Print and shaded views of the part. All mm, measured from the part's lowest x, y and z. Coordinates: 2 decimals unless noted, no trailing zeros. Order: outer loops, then holes, each group sorted by start corner. A loop starts at its lowest first (then second) coordinate and runs counter-clockwise, first axis right, second up. Notation, with made-up numbers: M -24,4.5 L 23,4.5 A27 cw 23,43.5 Z; hole C 2.25,9 d5. An arc over 180 degrees is marked long. Return JSON: item names as keys, results as strings.
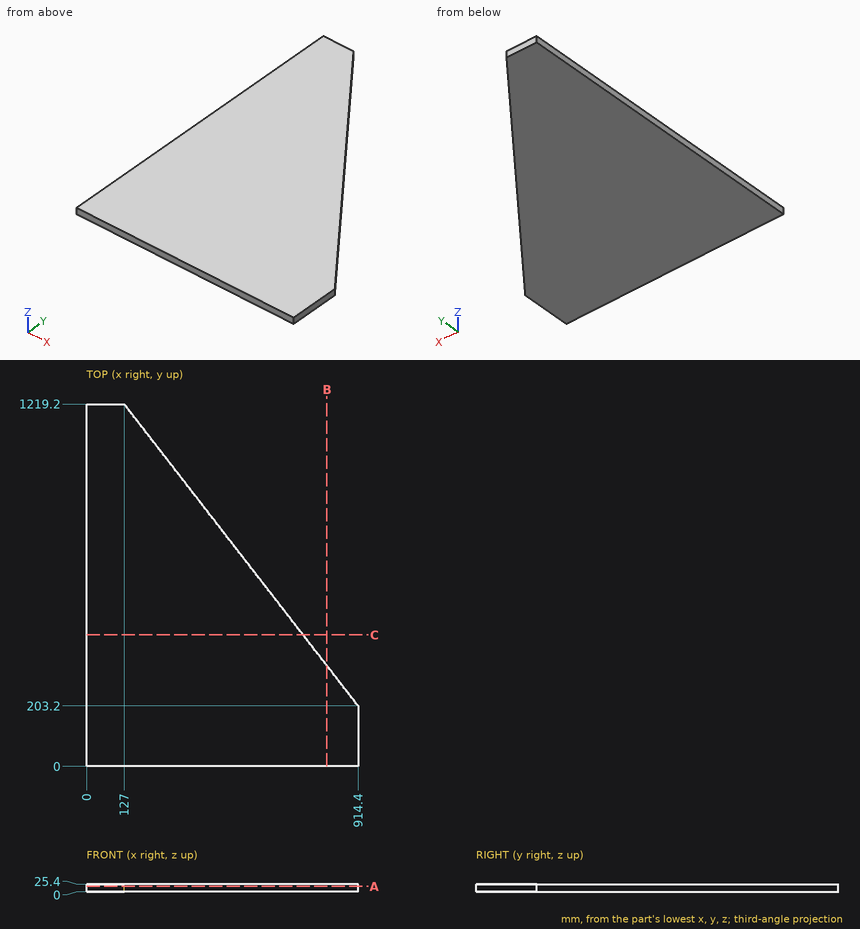
Item 1: Saw through at A-A (z = 18). Write the cut outline in (x, y).
Check result:
{"outline": "M 0,0 L 914.4,0 L 914.4,203.2 L 127,1219.2 L 0,1219.2 Z"}
Item 2: Saw through at C-C (y = 442). Write the cut outline in (x, z), and give its area (3 significant figures).
Check result:
{"outline": "M 0,0 L 729.33,0 L 729.33,25.4 L 0,25.4 Z", "area": "18,500 mm2"}
Item 3: Wall check: line 1 (X direction, y = 651, z = 18) (3 decimals); line 2 (Y direction, x = 215, z = 15.25); line 3 (Y direction, x = 523.5, z = 6.25). Give the ranges that are in metal, low to high.
Check result:
{"line 1": "x = 0 to 567.355", "line 2": "y = 0 to 1105.65", "line 3": "y = 0 to 707.59"}
Item 4: Drop flat-ended pins along their axis: pin 1 Ø10 at (x, z) = (500, 18.5) entering from +Y; pin 2 Ø12 at (y, z) = (490, 16.5) entering from +X. Give the stop position or say it passes through.
Check result:
{"pin 1": "stops at y = 744.36", "pin 2": "stops at x = 696.78"}
Item 5: Saw through at B-B (x = 809). Write the cut outline in (y, z).
Check result:
{"outline": "M 0,0 L 339.2,0 L 339.2,25.4 L 0,25.4 Z"}
